Model file for the job. Use its own axes, mm. A direction names the side the tool comes from. Give positions to 0.01 mm unless a question says otherwise; leave off trailing zeros. Loops run counter-clockwise (first coordinate to the right, second up) from the corner with the lowest first, then second, coordinate; pieces in that order, holes last. Notation, with made-up numbers: (-35.75, 54.5) - (-3.75, 54.5) arc R18 ccw to (-3.75, 81.5) - close; hole circle Ø1 at (76, 3.25). An arc over 180 degrees is marked (long way). Use a Markdown table: item, result.
Autodesk Fusion 360 part; units mm, degrees
sketch "Sketch1" plane through (0, 0, 0) normal (0, 1, 0) x (1, 0, 0)
  line L0 (0, 0) -> (66.6, 0)
  line L1 (66.6, 0) -> (66.6, -56.6)
  line L2 (66.6, -56.6) -> (0, -56.6)
  line L3 (0, -56.6) -> (0, 0)
  line L4 (0, 0) -> (-20, 0)
  line L5 (-20, 0) -> (-20, -10)
  line L6 (-20, -10) -> (-10, -10)
  line L7 (0, -10) -> (0, 0)
  line L8 (-10, -10) -> (-10, -66.6)
  line L9 (-10, -66.6) -> (0, -66.6)
  line L10 (0, -56.6) -> (0, -10)
  line L11 (0, -66.6) -> (66.6, -66.6)
  line L12 (66.6, -56.6) -> (0, -56.6)
  line L13 (66.6, -66.6) -> (76.6, -66.6)
  line L14 (76.6, -66.6) -> (76.6, -10)
  line L15 (76.6, 0) -> (66.6, 0)
  line L16 (66.6, 0) -> (66.6, -56.6)
  line L17 (66.6, 0) -> (86.6, 0)
  line L18 (86.6, 0) -> (86.6, -10)
  line L19 (86.6, -10) -> (76.6, -10)
  line L20 (66.6, -10) -> (66.6, 0)
  dimension "d19" = 66.6
  dimension "d20" = 56.6
  dimension "d21" = 20
  dimension "d22" = 10
  dimension "d23" = 10
  dimension "d24" = 56.6
  dimension "d25" = 10
  dimension "d26" = 20
  dimension "d27" = 10
extrude "Extrude2" add sketch "Sketch1" along normal blind 20.5 contours L1 L2 L3 L4 L5 L6 L7 L8 L9 L10 L11 L12 L13 L14 L15 L16 L17 L18 L19 L20
sketch "Sketch4" plane through (0, 0, 10) normal (0, 0, 1) x (-1, 0, 0)
  line L0 (20, 0) -> (10, 0)
  line L1 (10, 0) -> (10, -20.5)
  line L2 (10, -20.5) -> (20, -20.5)
  line L3 (20, -20.5) -> (20, 0)
  circle A0 centre (15, -10.25) radius 1.5
  dimension "d32" = 3
sketch "Sketch5" plane through (0, 0, 10) normal (0, 0, 1) x (-1, 0, 0)
  line L0 (-76.6, 0) -> (-86.6, 0)
  line L1 (-86.6, 0) -> (-86.6, -20.5)
  line L2 (-86.6, -20.5) -> (-76.6, -20.5)
  line L3 (-76.6, -20.5) -> (-76.6, 0)
  circle A0 centre (-81.6, -10.25) radius 1.5
  dimension "d33" = 3
hole "Hole2" at (-15, 10.25, 10) at (81.6, 10.25, 10) direction (0, 0, -1) diameter 2.529 depth 15 tip angle 118
sketch "Sketch6" plane through (0, 0, 0) normal (0, 0, -1) x (1, 0, 0)
  circle A0 centre (-15, -10.25) radius 1.2645
  line L0 (0, 0) -> (-20, 0)
  line L1 (-20, 0) -> (-20, -20.5)
  line L2 (-20, -20.5) -> (0, -20.5)
  line L3 (0, -20.5) -> (0, 0)
  line L4 (-20, 0) -> (0, 0)
  line L5 (0, 0) -> (0, -20.5)
  line L6 (0, -20.5) -> (-20, -20.5)
  line L7 (-20, -20.5) -> (-20, 0)
  line L8 (-15, -10.25) -> (-20, -10.25)
  line L9 (-15, -10.25) -> (-15, 0)
extrude "Extrude3" cut 1 faces at (18.8667, 6.8333, 66.6) along direction (0, 0, -1) blind 5
fillet "Fillet3" radius 5 2 edges at (-10, 10.25, 61.6) (76.6, 10.25, 61.6)
(1) Slice it at B-B, the plane y = 10.25. Write the cut outline in (x, z), plus the area to 3 significant figures.
Computed:
| item | result |
|---|---|
| outline | (-20, 0) - (-16.26, 0) - (-16.26, 10) - (-20, 10) - close; (-13.74, 0) - (0, 0) - (0, 56.6) - (66.6, 56.6) - (66.6, 0) - (80.34, 0) - (80.34, 10) - (76.6, 10) - (76.6, 56.6) arc R5 ccw to (71.6, 61.6) - (-5, 61.6) arc R5 ccw to (-10, 56.6) - (-10, 10) - (-13.74, 10) - close; (82.86, 0) - (86.6, 0) - (86.6, 10) - (82.86, 10) - close |
| area | 1,700 mm² |
(2) Mould opens along X. For faces 5 (the flat face through (77, 10, 0)), 6 (the cylindrical face through (75.1, 10.39, 60.17)), 7 (the cylindrical face through (-15.855, 11.182, 4.93)) say: pulls with the +X half, pulls with the -X half, needs draft (parallel to the pull), parting line crosses it, or undercut.
Computed:
| item | result |
|---|---|
| face 5 | needs draft |
| face 6 | pulls with the +X half |
| face 7 | undercut |
(3) Slice it at C-C, the plane x = -15. Write the cut outline in (y, z).
Computed:
| item | result |
|---|---|
| outline | (0, 0) - (8.99, 0) - (8.99, 10) - (0, 10) - close; (11.51, 0) - (20.5, 0) - (20.5, 10) - (11.51, 10) - close |
(4) Slice it at A-A, the plane z = 12. Write the cut outline in (x, y), plus the area to 3 significant figures.
Computed:
| item | result |
|---|---|
| outline | (-10, 0) - (0, 0) - (0, 20.5) - (-10, 20.5) - close; (66.6, 0) - (76.6, 0) - (76.6, 20.5) - (66.6, 20.5) - close |
| area | 410 mm² |
(5) Drill centre lines: probe 1 along X at (y, z) = (10.25, 6); probe 2 along X at (y, z) = (12.25, 20.5); probe 3 along X at (y, z) = (3, 8). Where is each one in solid material? Low to high. Write a range as [from, to].
Computed:
| item | result |
|---|---|
| probe 1 | [-20, -16.26], [-13.74, 0], [66.6, 80.34], [82.86, 86.6] |
| probe 2 | [-10, 0], [66.6, 76.6] |
| probe 3 | [-20, 0], [66.6, 86.6] |
(6) Slice it at D-D, the plane y = 16.5. Write the cut outline in (x, z), plus the area to 3 significant figures.
Computed:
| item | result |
|---|---|
| outline | (-20, 0) - (0, 0) - (0, 56.6) - (66.6, 56.6) - (66.6, 0) - (86.6, 0) - (86.6, 10) - (76.6, 10) - (76.6, 56.6) arc R5 ccw to (71.6, 61.6) - (-5, 61.6) arc R5 ccw to (-10, 56.6) - (-10, 10) - (-20, 10) - close |
| area | 1,750 mm² |
(7) 3-axis set-ups, long thin cutter, end or side, ignore diameter. For faces 1 (the flat face through (33, 10, 61.6)), 2 (the flat face through (34, 10, 56.6)), 3 (the flat face through (76.6, 10, 34)), 4 (the flat face through (-17, 10, 10)): which of +Z, -Z, +X, -X, +Y, -Y reach the whole face in a straight line?
Computed:
| item | result |
|---|---|
| face 1 | +Z, +X, -X, +Y, -Y |
| face 2 | -Z, +Y, -Y |
| face 3 | +Z, +X, +Y, -Y |
| face 4 | +Z, -X, +Y, -Y |
(8) Pin check, flat tips, straight feed: P1, Ø1, axis at y = 14, z = 39, coming from the +X side; P2, Ø10, axis at x = 7, z = 9.5, coming from the -Y side; P3, Ø5, axis at x = -17, y = 12, coming from the +Z side; P4, Ø4, axis at y = 14.5, z = 28.5, coming from the -X side. Stop position of each tip, or through.
Computed:
| item | result |
|---|---|
| P1 | x = 76.6 |
| P2 | through |
| P3 | z = 10 |
| P4 | x = -10 |
